The listing builds one solid part. Answer for the finished solid, in the listing's coordinates (mm). A direction names the side the tool comes from. Coordinates: 2 decimals unless noted, no trailing zeros. Order: outer loops, then holes, each group sorted by start corner. A loop starts at its lowest first (then second) coordinate and runs counter-clockwise, first axis right, second up. Notation, with made-up numbers: (27.25, 20.25) -> (75.25, 20.25) arc R24 ccw to (75.25, 53.25) -> close; hole circle Ø11 at (20, -11). An arc over 180 degrees is marked (long way). Put each result on its own line as item: value. Start each with the question number.
```python
from build123d import *

# Parameters (mm, degrees)
F1_DEPTH = 3.175
F3_DEPTH = 15.24
F4_W     = 1.27
F4_H     = 12.7
F4_W_2   = 12.7
F4_H_2   = 1.27
F5_DEPTH = 3.175
F6_SIZE  = 1.26999
F8_W     = 133.35
F8_H     = 69.85
F9_DEPTH = 6.35
F10_R    = 1.27
F11_R    = 1.27


# Not quite as in the source:
# - a fillet or chamfer is up to 0.001 mm smaller than in the source, because OpenCascade refuses the exact size


with BuildPart() as f1:
    # F0 (on Top) → F1 (new body)
    with BuildSketch(Plane.XY):
        with BuildLine():
            ThreePointArc((67.31, 32.385), (66.3800640303, 34.6300640303), (64.135, 35.56))
            Line((64.135, 35.56), (-64.135, 35.56))
            ThreePointArc((-64.135, 35.56), (-66.3800640303, 34.6300640303), (-67.31, 32.385))
            Line((-67.31, 32.385), (-67.31, -32.385))
            ThreePointArc((-67.31, -32.385), (-66.3800640303, -34.6300640303), (-64.135, -35.56))
            Line((-64.135, -35.56), (64.135, -35.56))
            ThreePointArc((64.135, -35.56), (66.3800640303, -34.6300640303), (67.31, -32.385))
            Line((67.31, -32.385), (67.31, 32.385))
        make_face()
        with BuildLine():
            Line((38.1, -1.905), (-38.1, -1.905))
            ThreePointArc((-38.1, -1.905), (-40.005, 0), (-38.1, 1.905))
            Line((-38.1, 1.905), (38.1, 1.905))
            ThreePointArc((38.1, 1.905), (40.005, 0), (38.1, -1.905))
        make_face(mode=Mode.SUBTRACT)
    extrude(amount=F1_DEPTH)

    # F2 (on Top) → F3 (join)
    with BuildSketch(Plane.XY):
        with BuildLine():
            Line((-67.31, -6.35), (-67.31, 6.35))
            Line((-67.31, 6.35), (-68.8975, 6.35))
            ThreePointArc((-68.8975, 6.35), (-71.1425640303, 5.4200640303), (-72.0725, 3.175))
            Line((-72.0725, 3.175), (-72.0725, -3.175))
            ThreePointArc((-72.0725, -3.175), (-71.1425640303, -5.4200640303), (-68.8975, -6.35))
            Line((-68.8975, -6.35), (-67.31, -6.35))
        make_face()
        with BuildLine():
            Line((-44.45, -37.1475), (-44.45, -35.56))
            Line((-44.45, -35.56), (-57.15, -35.56))
            Line((-57.15, -35.56), (-57.15, -37.1475))
            ThreePointArc((-57.15, -37.1475), (-56.2200640303, -39.3925640303), (-53.975, -40.3225))
            Line((-53.975, -40.3225), (-47.625, -40.3225))
            ThreePointArc((-47.625, -40.3225), (-45.3799359697, -39.3925640303), (-44.45, -37.1475))
        make_face()
        with BuildLine():
            Line((-57.15, 35.56), (-44.45, 35.56))
            Line((-44.45, 35.56), (-44.45, 37.1475))
            ThreePointArc((-44.45, 37.1475), (-45.3799359697, 39.3925640303), (-47.625, 40.3225))
            Line((-47.625, 40.3225), (-53.975, 40.3225))
            ThreePointArc((-53.975, 40.3225), (-56.2200640303, 39.3925640303), (-57.15, 37.1475))
            Line((-57.15, 37.1475), (-57.15, 35.56))
        make_face()
        with BuildLine():
            Line((57.15, -35.56), (44.45, -35.56))
            Line((44.45, -35.56), (44.45, -37.1475))
            ThreePointArc((44.45, -37.1475), (45.3799359697, -39.3925640303), (47.625, -40.3225))
            Line((47.625, -40.3225), (53.975, -40.3225))
            ThreePointArc((53.975, -40.3225), (56.2200640303, -39.3925640303), (57.15, -37.1475))
            Line((57.15, -37.1475), (57.15, -35.56))
        make_face()
        with BuildLine():
            Line((67.31, 6.35), (67.31, -6.35))
            Line((67.31, -6.35), (68.8975, -6.35))
            ThreePointArc((68.8975, -6.35), (71.1425640303, -5.4200640303), (72.0725, -3.175))
            Line((72.0725, -3.175), (72.0725, 3.175))
            ThreePointArc((72.0725, 3.175), (71.1425640303, 5.4200640303), (68.8975, 6.35))
            Line((68.8975, 6.35), (67.31, 6.35))
        make_face()
        with BuildLine():
            Line((44.45, 35.56), (57.15, 35.56))
            Line((57.15, 35.56), (57.15, 37.1475))
            ThreePointArc((57.15, 37.1475), (56.2200640303, 39.3925640303), (53.975, 40.3225))
            Line((53.975, 40.3225), (47.625, 40.3225))
            ThreePointArc((47.625, 40.3225), (45.3799359697, 39.3925640303), (44.45, 37.1475))
            Line((44.45, 37.1475), (44.45, 35.56))
        make_face()
    extrude(amount=F3_DEPTH)

    # F4 (on face) → F5 (join)
    with BuildSketch(Plane.XY.offset(15.24)):
        with BuildLine():
            Line((-68.8975, -6.35), (-67.31, -6.35))
            Line((-67.31, -6.35), (-67.31, 6.35))
            Line((-67.31, 6.35), (-68.8975, 6.35))
            ThreePointArc((-68.8975, 6.35), (-71.1425640303, 5.4200640303), (-72.0725, 3.175))
            Line((-72.0725, 3.175), (-72.0725, -3.175))
            ThreePointArc((-72.0725, -3.175), (-71.1425640303, -5.4200640303), (-68.8975, -6.35))
        make_face()
        with Locations((-66.675, 0)):
            Rectangle(F4_W, F4_H)
        with BuildLine():
            Line((-44.45, -35.56), (-57.15, -35.56))
            Line((-57.15, -35.56), (-57.15, -37.1475))
            ThreePointArc((-57.15, -37.1475), (-56.2200640303, -39.3925640303), (-53.975, -40.3225))
            Line((-53.975, -40.3225), (-47.625, -40.3225))
            ThreePointArc((-47.625, -40.3225), (-45.3799359697, -39.3925640303), (-44.45, -37.1475))
            Line((-44.45, -37.1475), (-44.45, -35.56))
        make_face()
        with Locations((-50.8, -34.925)):
            Rectangle(F4_W_2, F4_H_2)
        with BuildLine():
            Line((-57.15, 37.1475), (-57.15, 35.56))
            Line((-57.15, 35.56), (-44.45, 35.56))
            Line((-44.45, 35.56), (-44.45, 37.1475))
            ThreePointArc((-44.45, 37.1475), (-45.3799359697, 39.3925640303), (-47.625, 40.3225))
            Line((-47.625, 40.3225), (-53.975, 40.3225))
            ThreePointArc((-53.975, 40.3225), (-56.2200640303, 39.3925640303), (-57.15, 37.1475))
        make_face()
        with Locations((-50.8, 34.925)):
            Rectangle(F4_W_2, F4_H_2)
        with Locations((50.8, 34.925)):
            Rectangle(F4_W_2, F4_H_2)
        with BuildLine():
            Line((44.45, 35.56), (57.15, 35.56))
            Line((57.15, 35.56), (57.15, 37.1475))
            ThreePointArc((57.15, 37.1475), (56.2200640303, 39.3925640303), (53.975, 40.3225))
            Line((53.975, 40.3225), (47.625, 40.3225))
            ThreePointArc((47.625, 40.3225), (45.3799359697, 39.3925640303), (44.45, 37.1475))
            Line((44.45, 37.1475), (44.45, 35.56))
        make_face()
        with Locations((66.675, 0)):
            Rectangle(F4_W, F4_H)
        with BuildLine():
            Line((68.8975, 6.35), (67.31, 6.35))
            Line((67.31, 6.35), (67.31, -6.35))
            Line((67.31, -6.35), (68.8975, -6.35))
            ThreePointArc((68.8975, -6.35), (71.1425640303, -5.4200640303), (72.0725, -3.175))
            Line((72.0725, -3.175), (72.0725, 3.175))
            ThreePointArc((72.0725, 3.175), (71.1425640303, 5.4200640303), (68.8975, 6.35))
        make_face()
        with BuildLine():
            Line((57.15, -37.1475), (57.15, -35.56))
            Line((57.15, -35.56), (44.45, -35.56))
            Line((44.45, -35.56), (44.45, -37.1475))
            ThreePointArc((44.45, -37.1475), (45.3799359697, -39.3925640303), (47.625, -40.3225))
            Line((47.625, -40.3225), (53.975, -40.3225))
            ThreePointArc((53.975, -40.3225), (56.2200640303, -39.3925640303), (57.15, -37.1475))
        make_face()
        with Locations((50.8, -34.925)):
            Rectangle(F4_W_2, F4_H_2)
    extrude(amount=F5_DEPTH)

    # F6 (size 1.27 in the source; OpenCascade refuses exactly that, so slightly less here)
    f6_edges = [f1.edges().sort_by_distance(p)[0] for p in [
        (50.8, -34.29, 15.24),
        (50.8, -34.29, 18.415),
        (66.04, 0, 18.415),
        (50.8, 34.29, 18.415),
        (-50.8, -34.29, 18.415),
        (-66.04, 0, 18.415),
        (-50.8, 34.29, 18.415),
        (-66.04, 0, 15.24),
        (-50.8, -34.29, 15.24),
        (66.04, 0, 15.24),
        (50.8, 34.29, 15.24),
        (-50.8, 34.29, 15.24),
    ]]
    chamfer(f6_edges, length=F6_SIZE)

    # F8 (on face) → F9 (cut)
    with BuildSketch(Plane.XY.offset(18.415)):
        Rectangle(F8_W, F8_H)
    extrude(amount=-F9_DEPTH, mode=Mode.SUBTRACT)

    # F10
    f10_edges = [f1.edges().sort_by_distance(p)[0] for p in [
        (-50.8, -40.3225, 0),
        (-45.379936, -39.392564, 0),
        (-56.220064, -39.392564, 0),
        (0, -35.56, 0),
        (45.379936, -39.392564, 0),
        (56.220064, -39.392564, 0),
        (60.6425, -35.56, 0),
        (71.142564, -5.420064, 0),
        (67.31, 19.3675, 0),
        (56.220064, 39.392564, 0),
        (0, 35.56, 0),
        (-50.8, 40.3225, 0),
        (-60.6425, 35.56, 0),
        (-71.142564, 5.420064, 0),
        (-67.31, -19.3675, 0),
    ]]
    fillet(f10_edges, radius=F10_R)

    # F11
    f11_edges = [f1.edges().sort_by_distance(p)[0] for p in [
        (67.31, 0, 3.175),
        (-50.8, -35.56, 3.175),
        (50.8, -35.56, 3.175),
        (-67.31, 0, 3.175),
        (50.8, 35.56, 3.175),
        (-50.8, 35.56, 3.175),
    ]]
    fillet(f11_edges, radius=F11_R)


solid = f1.part
```
(1) The part is cut by section C-C on y = 26.5. Determine the outline of the cut face in (x, z) (3 decimals).
(2) The part is cut by section B-B on x = -9.5. Determine the outline of the cut face in (y, z) (3 decimals), plus the area to 3 significant figures.
(3) A tool of negligible diameter and unlimited length cuts with its end or side. For faces 4 (the flat face through (51, -35.56, 10)), 5 (the cylindrical face through (-45.405, -39.417, 9.722)), 6 (the cylindrical face through (-40.005, -0.042, 1.565)), 7 (the cylindrical face through (-45.36, 39.37, 9.72)), from which of +Z, -Z, +X, -X, +Y, -Y can it reach the whole face along a straight path? Write none if from no direction.
(4) Find the intervals of material crossed by L1, parallel to Y at x = 18.5, z = 1.5 (3 decimals); L2, parallel to Y at x = 49, z = 11.25; L3, parallel to Z at x = -8, y = -25 (3 decimals), in increasing order.
(5) Each of these flat-tipped pins is pushed along its axis until it touches: P1, Ø6, axis at x = 4.5, z = 8.5, coming from the +Y side (3 decimals); P2, Ø3, axis at y = -35, z = 8, coming from the -X side; P3, Ø1.4, axis at x = 68, z = 11, coming from the +Y side; P4, Ø3.5, axis at x = -5.5, z = 1.5, coming from the +Y side. Where does it stop, or does it pass through?
(6) For a pull along Z with two mould halves and no side action, classify faces 1 (the cylindrical face through (40.005, 0.042, 1.565)), 2 (the flat face through (-1, -8, 0)), 3 (the flat face through (-51, 35.56, 10)) as released by +Z, released by -Z, zero draft, split by the parting line, or undercut.
Worked out:
1. outline: (-67.31, 1.27) arc R1.27 ccw to (-66.04, 0) -> (66.04, 0) arc R1.27 ccw to (67.31, 1.27) -> (67.31, 3.175) -> (-67.31, 3.175) -> close
2. outline: (-35.56, 1.27) arc R1.27 ccw to (-34.29, 0) -> (-1.905, 0) -> (-1.905, 3.175) -> (-35.56, 3.175) -> close; (1.905, 0) -> (34.29, 0) arc R1.27 ccw to (35.56, 1.27) -> (35.56, 3.175) -> (1.905, 3.175) -> close
2. area: 213 mm2
3. face 4: +X, -X
3. face 5: +Z, -Z, -Y
3. face 6: +Z, -Z
3. face 7: +Z, -Z, +Y
4. L1: -35.56 to -1.905, 1.905 to 35.56
4. L2: -40.32 to -35.56, 35.56 to 40.32
4. L3: 0 to 3.175
5. P1: through
5. P2: x = -57.15
5. P3: y = 6.35
5. P4: y = 35.56
6. face 1: zero draft
6. face 2: released by -Z
6. face 3: undercut
